Job drawing, mm, ordinate dimensions from the low corner. One solid piece. Give positions to 0.01 mm unless a question says otherwise; leave off trailing zeros. Write each loop counter-clockwise with the first axis right and the second up, starting at its lowest first coordinate (ties: lowest second). Pieces come first, ordered by that corner, then holes. Notation, with made-up numbers: M 73,15.25 L 113,15.25 A23 cw 113,29.25 Z; hole C 49,-15.75 d8. An arc over 180 degrees is marked long. Use a Markdown table: item, result.
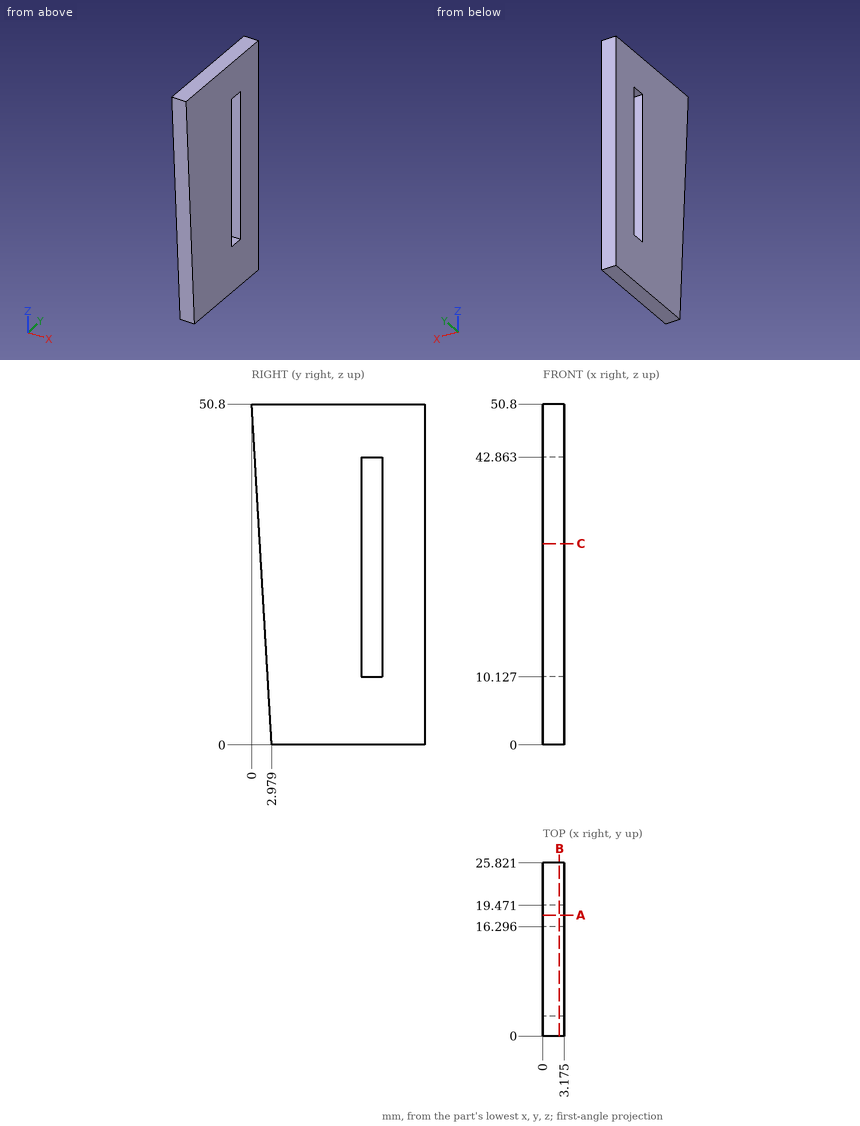
1. Drop a flat-ended pin along its axis: P1, Ø1.5, axis at x = 1, z = 9, coming from the -Y side. Give the stop position or say it passes through.
Findings below:
| item | result |
|---|---|
| P1 | y = 2.41 |
2. Drill centre lines: L1, parallel to Z at x = 2.4, y = 17; L2, parallel to Y at x = 1.15, z = 34 (1 decimal); L3, parallel to Y at x = 2.1, z = 27.5 (1 decimal). Where is each one in solid material? Low to high.
Findings below:
| item | result |
|---|---|
| L1 | 0 to 10.13, 42.86 to 50.8 |
| L2 | 1 to 16.3, 19.5 to 25.8 |
| L3 | 1.4 to 16.3, 19.5 to 25.8 |
3. Cut at B-B, the plane x = 2.45. Give the cut face in (y, z), then the cut area to 3 significant figures.
Findings below:
| item | result |
|---|---|
| outline | M 0,50.8 L 2.98,0 L 25.82,0 L 25.82,50.8 Z; hole M 16.3,10.13 L 19.47,10.13 L 19.47,42.86 L 16.3,42.86 Z |
| area | 1,130 mm2 |
4. Cut at C-C, the plane z = 30. Give the cut face in (x, y) (1 decimal).
Findings below:
| item | result |
|---|---|
| outline | M 0,1.2 L 3.2,1.2 L 3.2,16.3 L 0,16.3 Z; M 0,19.5 L 3.2,19.5 L 3.2,25.8 L 0,25.8 Z |
5. Cut at A-A, the plane y = 18. Give the cut face in (x, z) (1 decimal).
Findings below:
| item | result |
|---|---|
| outline | M 0,0 L 3.2,0 L 3.2,10.1 L 0,10.1 Z; M 0,42.9 L 3.2,42.9 L 3.2,50.8 L 0,50.8 Z |
